Autodesk Inventor part; units mm, degrees
ref_plane "YZ Plane" through (0, 0, 0) normal (1, 0, 0) x (0, 1, 0)
ref_plane "XZ Plane" through (0, 0, 0) normal (0, 1, 0) x (-1, 0, 0)
ref_plane "XY Plane" through (0, 0, 0) normal (0, 0, 1) x (1, 0, 0)
sketch "Эскиз1" plane through (0, 0, 0) normal (0, 1, 0) x (-1, 0, 0)
  line L0 (0, 0) -> (50, 0)
  line L1 (50, 0) -> (50, -50)
  line L2 (50, -50) -> (0, -50)
  line L3 (0, -50) -> (0, 0)
  line L4 (3, -47) -> (47, -47)
  line L5 (47, -47) -> (47, -3)
  line L6 (47, -3) -> (3, -3)
  line L7 (3, -3) -> (3, -47)
  dimension "d0" = 50
  dimension "d1" = 50
  dimension "d2" = 3
extrude "Выдавливание1" add sketch "Эскиз1" along normal blind 350
sketch "Эскиз2" plane through (-50, 0, 0) normal (0, 0, 1) x (1, 0, 0)
  line L0 (0, 0) -> (50, 0)
  line L1 (50, 0) -> (50, 350)
  line L2 (0, 350) -> (50, 350)
  line L3 (0, 0) -> (0, 350)
  circle A0 centre (43.95, 325) radius 3.05
  circle A1 centre (43.95, 275) radius 3.05
  circle A2 centre (6.05, 325) radius 3.05
  circle A3 centre (6.05, 275) radius 3.05
  line L4 (3, 0) -> (47, 0)
  line L5 (47, 0) -> (47, 350)
  line L6 (3, 350) -> (47, 350)
  line L7 (3, 0) -> (3, 350)
  circle A4 centre (6.05, 35) radius 3.05
  circle A5 centre (43.95, 35) radius 3.05
  circle A6 centre (43.95, 75) radius 3.05
  circle A7 centre (6.05, 75) radius 3.05
  dimension "d5" = 6.1
  dimension "d8" = 50
  dimension "d11" = 37.9
  dimension "d14" = 25
  dimension "d15" = 6.05
  dimension "d18" = 6.1
  dimension "d19" = 35
  dimension "d22" = 40
extrude "Выдавливание2" cut sketch "Эскиз2" against normal through all contours A5 | A6 | A1 | A0 | A2 | A3 | A7 | A4
equation "\"d0\" = width_profile_femur"
equation "\"d1\" = hight_profile_femur"
equation "\"d2\" = thickness_profile_femur"
equation "\"d3\" = length_profile_femur"
equation "\"d5\" = d_main_screw_holes"
equation "\"d11\" = -2 * thickness_profile_femur + hight_profile_femur - d_main_screw_holes"
equation "\"d15\" = 0.5 * d_main_screw_holes + thickness_profile_femur"
equation "\"d18\" = d_main_screw_holes"
equation "\"tolerance_plazma\" = 0.1"
equation "\"thickness_steel\" = 3"
equation "\"d_main_screw_holes\" = 6.1"
equation "\"thickness_profile_tibea\" = 3"
equation "\"hight_shaft_shift\" = 37"
equation "\"thickness_profile_femur\" = 3"
equation "\"width_profile_femur\" = 50"
equation "\"width_shaft_shift\" = 35"
equation "\"length_profile_femur\" = 350"
equation "\"hight_profile_femur\" = 50"
equation "\"width_flattened_surface\" = 12"
properties part number "femur_profile"
Here's how the part is built. I have some questions about the finished solid (model axes, mm). A direction names the side the tool comes from. Round coordinates to 2 decimals unless told otherwise and drop trailing zeros. Loops run counter-clockwise (first coordinate to the right, second up) from the corner with the lowest first, then second, coordinate; pieces in that order, holes last. Notation, with made-up numbers: (86, 61.25) -> (107, 61.25) arc R31 cw to (107, 88.25) -> close; hole circle Ø11 at (48.5, 51.5). An arc over 180 degrees is marked (long way). Answer as CSV lines item,"result".
1. If we section it at D-D on x = -6.05: Count the separate pieces of the cut face and the enclosed holes in it, plus the area to 3 significant figures.
Final values:
separate pieces,"10"
enclosed holes,"0"
area,"1,950 mm^2"
2. If we section it at A-A on x = -24: Please give me the cut outline in (y, z), plus the area to 3 significant figures.
Final values:
outline,"(0, -50) -> (350, -50) -> (350, -47) -> (0, -47) -> close; (0, -3) -> (350, -3) -> (350, 0) -> (0, 0) -> close"
area,"2,100 mm^2"
3. Which directions (+Z, -Z, +X, -X, +Y, -Y) give clear straight access to the entire face, cutting with the end or side of a thin tool? Please do faces 1 (the face through (-6.711, 32.023, -1.479)), 2 (the face through (-47, 173, -25)).
Final values:
face 1,"+Z, -Z"
face 2,"+Y, -Y"
4. If I drill on L1, parallel to Y at x = -6, z = -49; L2, parallel to X at y = 275, z = -48; L3, parallel to Z at x = -10.5, y = 153, over which ranges is the centre line in solid material (lowest first)?
Final values:
L1,"y = 0 to 31.95, 38.05 to 71.95, 78.05 to 271.95, 278.05 to 321.95, 328.05 to 350"
L2,"x = -50 to -47, -40.9 to -9.1, -3 to 0"
L3,"z = -50 to -47, -3 to 0"
5. For pin 1 (5.5 mm diameter, centred on x = -43.95, y = 275, fed in from -Z), with a flat end and sliding along its axis, tell me the tip position at first contact or that it passes through.
Final values:
pin 1,"passes through"
6. If we section it at B-B on y = 106: Please give me the cut outline in (x, z), plus the area to 3 significant figures.
Final values:
outline,"(-50, -50) -> (0, -50) -> (0, 0) -> (-50, 0) -> close; hole (-47, -47) -> (-3, -47) -> (-3, -3) -> (-47, -3) -> close"
area,"564 mm^2"
7. Thinking about a two-plate mould opening in Y: for faces 3 (the face through (-2.7, 0, -24.9)), 4 (the face through (-6.711, 32.023, -48.479)), 5 (the face through (-25, 173, -47)), which applies, released by +Y, released by -Y, zero draft, split by the parting line, or undercut?
Final values:
face 3,"released by -Y"
face 4,"undercut"
face 5,"zero draft"
8. If we section it at C-C on z = -22: Please give me the cut outline in (x, y), plus the area to 3 significant figures.
Final values:
outline,"(-50, 0) -> (-47, 0) -> (-47, 350) -> (-50, 350) -> close; (-3, 0) -> (0, 0) -> (0, 350) -> (-3, 350) -> close"
area,"2,100 mm^2"
